Here's the drawing with two shaded views (mm, measured from the low corner). I have some questions. A direction names the side the tool comes from. Coordinates: 2 decimals unless noted, no trailing zeros. Order: outer loops, then holes, each group sorted by start corner. A loop starts at its lowest first (then second) coordinate and runs counter-clockwise, first axis right, second up. Notation, with made-up numbers: (-1, 13) - (55, 13) arc R23 ccw to (55, 44) - close; hole circle Ø5 at (55.25, 35.5). An arc over 180 degrees is marked (long way). Answer as a JSON object with one key per item and string values. Group by question number.
(1) We'd pull the mould along Z, two halves only. Please class the marked faces 1, 2, 3 and 4: pulls with the +Z half, pulls with the -Z half, needs draft (parallel to the pull), parting line crosses it, or undercut.
(2) Imagine slicing it at A-A, the plane z = 32.5. Write out the boundary of the cut face in (x, y), and give its area (3 significant figures).
(3) Imagine slicing it at C-C, the plane y = 11.5. Write out the boundary of the cut face in (x, z).
(4) Imagine slicing it at D-D, the plane z = 12. Write out the boundary of the cut face in (x, y), and give its area (3 significant figures).
(5) Imagine slicing it at B-B, the plane x = 7. Write out the boundary of the cut face in (y, z).
(6) Which directions (+Z, -Z, +X, -X, +Y, -Y) give clear straight access to the entire face, cutting with the end or side of a thin tool? Please do the marked faces 5, 6 and 7.
(7) Please list where these lines run through material, in increasing order: probe 1 along Z at (x, y) = (26.75, 13); probe 2 along X at (y, z) = (20, 28); probe 3 along Z at (x, y) = (15.5, 15.5).
(8) Will these pins go through, and if not, where does the flat tip stop? P1, Ø3, axis at x = 13.5, z = 48.5, coming from the +Y side; P2, Ø13.5, axis at x = 23, y = 29.5, coming from the +Z side; P3, Ø10, axis at y = 36, z = 18, coming from the +X side.
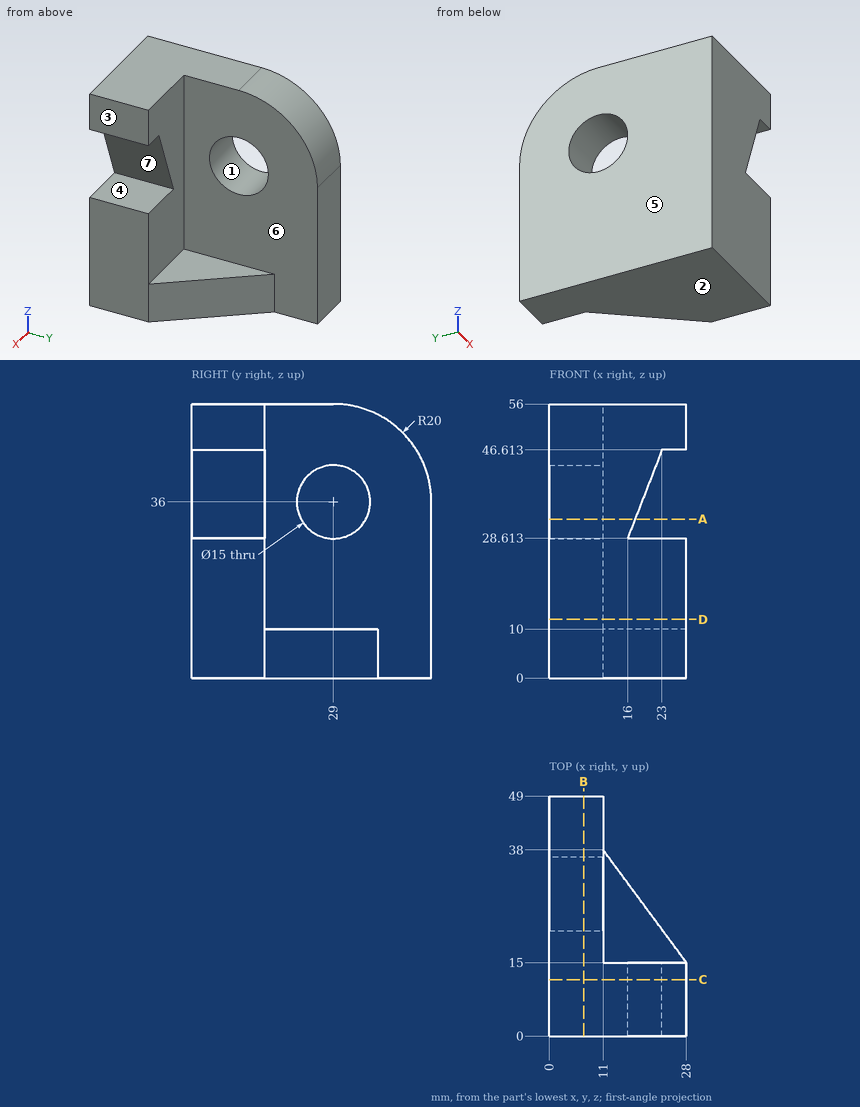
Result set:
{
 "1": {"face 1": "undercut", "face 2": "pulls with the -Z half", "face 3": "needs draft", "face 4": "undercut"},
 "2": {"outline": "(0, 0) - (17.51, 0) - (17.51, 15) - (11, 15) - (11, 22.37) - (0, 22.37) - close; (0, 35.63) - (11, 35.63) - (11, 49) - (0, 49) - close", "area": "491 mm^2"},
 "3": {"outline": "(0, 0) - (28, 0) - (28, 28.61) - (16, 28.61) - (23, 46.61) - (28, 46.61) - (28, 56) - (0, 56) - close"},
 "4": {"outline": "(0, 0) - (28, 0) - (28, 15) - (11, 15) - (11, 49) - (0, 49) - close", "area": "794 mm^2"},
 "5": {"outline": "(0, 0) - (49, 0) - (49, 36) arc R20 ccw to (29, 56) - (0, 56) - close; hole circle Ø15 at (29, 36)"},
 "6": {"face 5": "+Z, -Z, -X, +Y, -Y", "face 6": "+Z, +X, +Y", "face 7": "+X, +Y, -Y"},
 "7": {"probe 1": "z = 0 to 28.61, 46.61 to 56", "probe 2": "x = 0 to 11", "probe 3": "z = 0 to 10"},
 "8": {"P1": "stops at y = 15", "P2": "stops at z = 10", "P3": "stops at x = 11"}
}
